Read the model definition and answer for the solid it produces. Units are mm, in the model's axes. Face numbers are marked on the shaded views. A direction names the side the tool comes from. Coordinates: 2 decimals unless noted, no trailing zeros. Write each loop counter-clockwise with the first axis right and the second up, starting at its lowest first coordinate (ties: lowest second). Pieces come first, ordered by that corner, then holes. Notation, with made-up numbers: M 55,-21.5 L 105,-21.5 A23 ccw 105,3.5 Z; hole C 29,20 d3. An arc over 180 degrees is marked long. Write item = value, one per line.
from build123d import *

# Parameters (mm, degrees)
BOSS_EXTRUDE14_DEPTH    = 2.54
BOSS_EXTRUDE15_DEPTH    = 17.78
FILLET3_R               = 2.54
SKETCH5_R               = 1.905
CUT_EXTRUDE3_DEPTH      = 26.4
CUT_EXTRUDE3_DEPTH_BACK = 1
SKETCH6_W               = 3.81
SKETCH6_H               = 11.43
CUT_EXTRUDE4_DEPTH      = 26.4
CUT_EXTRUDE4_DEPTH_BACK = 1


with BuildPart() as part:
    # Sketch3 → Boss-Extrude14 (new body)
    with BuildSketch(Plane(origin=(0, 0, 0), x_dir=(1, 0, 0), z_dir=(0, 1, 0))):
        with BuildLine():
            Line((0, 62.41624918), (0, 0))
            Line((0, 0), (20.870167944, 0))
            Line((20.870167944, 0), (20.870167944, 10.900407257))
            ThreePointArc((20.870167944, 10.900407257), (4.064, 31.75), (20.870167944, 52.599592743))
            Line((20.870167944, 52.599592743), (20.870167944, 62.41624918))
            Line((20.870167944, 62.41624918), (0, 62.41624918))
        make_face()
    extrude(amount=BOSS_EXTRUDE14_DEPTH)

    # Sketch3<18> → Boss-Extrude15 (add)
    with BuildSketch(Plane(origin=(0, 0, 0), x_dir=(1, 0, 0), z_dir=(0, 1, 0))):
        with BuildLine():
            Line((20.870167944, 10.900407257), (20.870167944, 0))
            Line((20.870167944, 0), (25.4, 0))
            Line((25.4, 0), (25.4, 12.446))
            ThreePointArc((25.4, 12.446), (6.096, 31.75), (25.4, 51.054))
            Line((25.4, 51.054), (25.4, 62.41624918))
            Line((25.4, 62.41624918), (20.870167944, 62.41624918))
            Line((20.870167944, 62.41624918), (20.870167944, 52.599592743))
            ThreePointArc((20.870167944, 52.599592743), (4.064, 31.75), (20.870167944, 10.900407257))
        make_face()
    extrude(amount=BOSS_EXTRUDE15_DEPTH)

    # Fillet3
    fillet3_edges = [part.edges().sort_by_distance(p)[0] for p in [
        (20.870167944, 2.54, -57.507920962),
        (20.870167944, 2.54, -5.450203629),
        (4.064, 2.54, -31.75),
    ]]
    fillet(fillet3_edges, radius=FILLET3_R)

    # Sketch5 → Cut-Extrude3 (cut, two sides)
    with BuildSketch(Plane(origin=(0, 0, 0), x_dir=(0, 0, -1), z_dir=(1, 0, 0))) as cut_extrude3_sk:
        with Locations((6.5405, 11.43)):
            Circle(SKETCH5_R)
        with Locations((56.41762459, 11.43)):
            Circle(SKETCH5_R)
    extrude(amount=CUT_EXTRUDE3_DEPTH, mode=Mode.SUBTRACT)
    extrude(cut_extrude3_sk.sketch, amount=-CUT_EXTRUDE3_DEPTH_BACK, mode=Mode.SUBTRACT)

    # Sketch6 → Cut-Extrude4 (cut, two sides)
    with BuildSketch(Plane(origin=(0, 0, 0), x_dir=(0, 0, -1), z_dir=(1, 0, 0))) as cut_extrude4_sk:
        with Locations((25.273, 12.065)):
            Rectangle(SKETCH6_W, SKETCH6_H)
    extrude(amount=CUT_EXTRUDE4_DEPTH, mode=Mode.SUBTRACT)
    extrude(cut_extrude4_sk.sketch, amount=-CUT_EXTRUDE4_DEPTH_BACK, mode=Mode.SUBTRACT)


solid = part.part
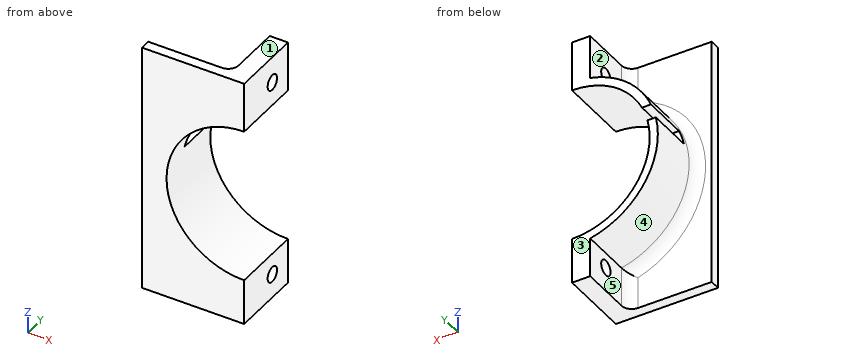
Item 1: Find section C-C (y = 11.43). Determine the outline of the cut face in (x, z), and give its area (3 significant figures).
Worked answers:
outline = M 4.56,-27.18 A21.34 ccw 20.87,-52.6 L 20.87,-54.51 L 25.4,-54.51 L 25.4,-51.05 A19.3 cw 6.65,-27.18 Z; M 5.78,-23.37 L 8.01,-23.37 A19.3 cw 25.4,-12.45 L 25.4,-8.45 L 20.87,-8.45 L 20.87,-10.9 A21.34 ccw Z; M 20.87,-62.42 L 25.4,-62.42 L 25.4,-58.32 L 20.87,-58.32 Z; M 20.87,-4.64 L 25.4,-4.64 L 25.4,0 L 20.87,0 Z
area = 178 mm²
Item 2: Find section B-B (z = -31.75). Determine the outline of the cut face in (x, y), and give its area (3 significant figures).
Worked answers:
outline = M 0,0 L 6.1,0 L 6.1,17.78 L 4.06,17.78 L 4.06,5.08 A2.54 cw 1.52,2.54 L 0,2.54 Z
area = 47.8 mm²
Item 3: Which of the six approach directions +Z, -Z, +X, -X, +Y, -Y give full straight-line access (tool end or side, diameter ignored) to the marked faces 1, 2, 3, 4 and 5?
Worked answers:
face_1 = +Z, +X, -X, +Y, -Y
face_2 = +Z, -X, +Y
face_3 = +Z, -Z, +X, -X, +Y
face_4 = -X, +Y
face_5 = -Z, -X, +Y
Item 4: Find section A-A (y = 14). Determine the outline of the cut face in (x, z), and give its area (3 significant figures).
Worked answers:
outline = M 4.56,-27.18 A21.34 ccw 20.87,-52.6 L 20.87,-62.42 L 25.4,-62.42 L 25.4,-51.05 A19.3 cw 6.65,-27.18 Z; M 5.78,-23.37 L 8.01,-23.37 A19.3 cw 25.4,-12.45 L 25.4,0 L 20.87,0 L 20.87,-10.9 A21.34 ccw Z
area = 212 mm²
Item 5: Consider line 1 along Z through (x, y) = (23.9, 11.43); line 2 along Z through (x, y) = (21.5, 12); line 3 along Y through (x, z) = (7.5, -16). Determine where each line is inside the solid, lowest interval first. Write a range as from..to.
Worked answers:
line_1 = -62.42..-58.32, -54.51..-51, -12.5..-8.45, -4.64..0
line_2 = -62.42..-58.24, -54.6..-50.66, -12.84..-8.36, -4.72..0
line_3 = 0..2.54
Item 6: Flat-ended cylindrical pins translate along their axes: pin 1 (3 mm diameter, centred on y = 8.5, z = -57.5, fed in from -X); pin 2 (5 mm diameter, centred on x = 18.5, y = 11, fed in from -Z); pin 3 (1 mm diameter, centred on y = 11.5, z = -36, fed in from -X); pin 4 (3 mm diameter, centred on x = 6.5, z = -25.5, fed in from +Y). Find the tip coordinate at first contact, or state that the pin passes through.
Worked answers:
pin_1 = 20.87
pin_2 = -62.42
pin_3 = 4.4
pin_4 = 6.35
